Autodesk Inventor part; units mm, degrees
ref_plane "YZ Plane" through (0, 0, 0) normal (1, 0, 0) x (0, 1, 0)
ref_plane "XZ Plane" through (0, 0, 0) normal (0, 1, 0) x (-1, 0, 0)
ref_plane "XY Plane" through (0, 0, 0) normal (0, 0, 1) x (1, 0, 0)
sketch "Sketch1" plane through (0, 0, 0) normal (0, 1, 0) x (-1, 0, 0)
  line L0 (0, 0) -> (0, -35)
  line L1 (0, -35) -> (37, -35)
  line L2 (37, -35) -> (37, -55)
  line L3 (37, -55) -> (48, -55)
  line L4 (48, -55) -> (48, 0)
  line L5 (48, 0) -> (22, 0)
  line L6 (22, 0) -> (22, 0)
  line L7 (22, 0) -> (0, 0)
  dimension "d0" = 35
  dimension "d1" = 37
  dimension "d2" = 20
  dimension "d3" = 11
  dimension "d4" = 55
  dimension "d5" = 26
  dimension "d6" = 0
extrude "Extrusion1" add sketch "Sketch1" along normal blind 50
shell "Shell1" thickness 5 removed faces 3 at (-48, 16.6667, -36.6667) at (-19.6667, 0, -23.3333) at (-19.6667, 50, -23.3333)
sketch "Sketch2" plane through (0, 0, 0) normal (1, 0, 0) x (0, 0, -1)
  line L0 (5, 0) -> (30, 0)
  line L1 (5, 0) -> (19, 0)
  line L2 (19, 0) -> (19, 17)
  line L3 (19, 17) -> (5, 17)
  line L4 (5, 17) -> (5, 0)
  point P0 (0, 0)
  dimension "d10" = 17
  dimension "d11" = 0
  dimension "d12" = 11
extrude "Extrusion2" cut sketch "Sketch2" against normal blind 10
sketch "Sketch3" plane through (-48, 0, -55) normal (-1, 0, 0) x (0, 0, 1)
  line L0 (0, 0) -> (0, 50)
  line L1 (5, 50) -> (25, 50)
  line L2 (0, 0) -> (5, 0)
  line L3 (5, 0) -> (5, 50)
  line L4 (5, 50) -> (0, 50)
  line L5 (0, 50) -> (0, 0)
  point P0 (55, 0)
extrude "Extrusion3" add sketch "Sketch3" along normal blind 15
sketch "Sketch4" plane through (-48, 0, 0) normal (-1, 0, 0) x (0, 0, 1)
  line L0 (-5, 0) -> (0, 0)
  line L1 (-5, 0) -> (-5, 50)
  line L2 (0, 0) -> (-5, 0)
  line L3 (-5, 0) -> (-5, 50)
  line L4 (-5, 50) -> (0, 50)
  line L5 (0, 50) -> (0, 0)
  point P0 (0, 0)
extrude "Extrusion4" add sketch "Sketch4" along normal blind 15
sketch "Sketch5" plane through (0, 17, -5) normal (0, 0, -1) x (-1, 0, 0)
  circle A0 centre (11.5, -8.5) radius 2.0828
  line L0 (63, -17) -> (0, -17)
  line L1 (0, -17) -> (0, 0)
  dimension "d19" = 4.1656
  dimension "d20" = 8.5
  dimension "d21" = 11.5
extrude "Extrusion5" cut sketch "Sketch5" against normal blind 15
sketch "Sketch6" plane through (0, 17, -5) normal (0, 0, -1) x (-1, 0, 0)
  circle A0 centre (28.505, 18.46) radius 2.0828
  line L0 (63, -17) -> (0, -17)
  line L1 (5, 0) -> (5, 33)
  dimension "d24" = 4.1656
  dimension "d25" = 35.46
  dimension "d26" = 23.505
extrude "Extrusion6" cut sketch "Sketch6" against normal blind 15
sketch "Sketch7" plane through (0, 17, -5) normal (0, 0, -1) x (-1, 0, 0)
  circle A0 centre (58.5, 19) radius 2.0828
  line L0 (63, 33) -> (63, -17)
  line L1 (5, 33) -> (63, 33)
  point P0 (0, -17)
  dimension "d29" = 4.1656
  dimension "d30" = 4.5
  dimension "d31" = 14
extrude "Extrusion7" cut sketch "Sketch7" against normal blind 15
sketch "Sketch13" plane through (0, 0, -35) normal (0, 0, -1) x (-1, 0, 0)
  circle A0 centre (11.5, 8.5) radius 2.0828
  line L0 (0, 0) -> (37, 0)
  line L1 (0, 0) -> (0, 50)
  dimension "d41" = 4.1656
  dimension "d42" = 8.5
  dimension "d43" = 11.5
extrude "Extrusion9" cut sketch "Sketch13" against normal blind 15
sketch "Sketch14" plane through (-37, 0, -55) normal (0, 0, -1) x (-1, 0, 0)
  circle A0 centre (-8.495, 35.46) radius 2.0828
  line L0 (-37, 0) -> (-37, 50)
  line L1 (0, 0) -> (26, 0)
  dimension "d46" = 4.1656
  dimension "d47" = 28.505
  dimension "d48" = 35.46
extrude "Extrusion10" cut sketch "Sketch14" against normal blind 15
sketch "Sketch15" plane through (-37, 0, -55) normal (0, 0, -1) x (-1, 0, 0)
  circle A0 centre (21.5, 36) radius 2.0828
  line L0 (0, 0) -> (26, 0)
  line L1 (26, 50) -> (26, 0)
  point P0 (-37, 0)
  dimension "d51" = 4.1656
  dimension "d52" = 36
  dimension "d53" = 4.5
extrude "Extrusion11" cut sketch "Sketch15" against normal blind 15
sketch "Sketch16" plane through (-42, 0, -30) normal (-1, 0, 0) x (0, 0, 1)
  line L0 (0, 0) -> (-5, 0)
  line L1 (-5, 0) -> (-5, 50)
  line L2 (-5, 50) -> (0, 50)
  line L3 (0, 50) -> (0, 0)
  point P0 (30, 0)
  dimension "d56" = 5
  dimension "d57" = 50
extrude "Extrusion12" add sketch "Sketch16" along normal blind 21
sketch "Sketch17" plane through (-5, 0, -30) normal (0, 0, 1) x (1, 0, 0)
  circle A0 centre (-23.505, 35.46) radius 2.0828
  line L0 (0, 0) -> (0, 50)
  line L1 (0, 0) -> (-58, 0)
  point P0 (5, 0)
  dimension "d60" = 4.1656
  dimension "d61" = 23.505
  dimension "d62" = 35.46
extrude "Extrusion13" cut sketch "Sketch17" against normal blind 10
sketch "Sketch18" plane through (-42, 0, -35) normal (0, 0, -1) x (-1, 0, 0)
  circle A0 centre (16.5, 36) radius 2.0828
  line L0 (21, 50) -> (21, 0)
  line L1 (0, 0) -> (21, 0)
  point P0 (-42, 0)
  dimension "d65" = 4.1656
  dimension "d67" = 36
  dimension "d70" = 4.5
extrude "Extrusion14" cut sketch "Sketch18" against normal blind 10
sketch "Sketch20" plane through (-63, 0, 0) normal (-1, 0, 0) x (0, 0, 1)
  line L0 (0, 0) -> (-5, 0)
  line L1 (-5, 17) -> (-5, 50)
  line L2 (0, 0) -> (-5, 0)
  line L3 (-5, 0) -> (-5, 50)
  line L4 (-5, 50) -> (0, 50)
  line L5 (0, 50) -> (0, 0)
extrude "Extrusion15" add sketch "Sketch20" along normal blind 2.583
sketch "Sketch21" plane through (-63, 0, -30) normal (-1, 0, 0) x (0, 0, 1)
  line L0 (-20, 50) -> (-5, 50)
  line L1 (11, 0) -> (0, 0)
  line L2 (-5, 50) -> (0, 50)
  line L3 (0, 50) -> (0, 0)
  line L4 (0, 0) -> (-5, 0)
  line L5 (-5, 0) -> (-5, 50)
  point P0 (30, 0)
extrude "Extrusion16" add sketch "Sketch21" along normal blind 2.583
sketch "Sketch22" plane through (-63, 0, -55) normal (-1, 0, 0) x (0, 0, 1)
  line L0 (0, 0) -> (0, 50)
  line L1 (5, 0) -> (5, 50)
  line L2 (0, 50) -> (5, 50)
  line L3 (5, 50) -> (5, 0)
  line L4 (5, 0) -> (0, 0)
  line L5 (0, 0) -> (0, 50)
  point P0 (55, 0)
extrude "Extrusion17" add sketch "Sketch22" along normal blind 2.583
sketch "Sketch23" plane through (0, 0, 0) normal (0, 0, 1) x (1, 0, 0)
  line L0 (0, 50) -> (-37, 50)
  line L1 (-65.583, 50) -> (-65.583, 0)
  line L2 (0, 50) -> (-65.583, 50)
  line L3 (-65.583, 50) -> (-65.583, 43.083)
  line L4 (-65.583, 43.083) -> (0, 43.083)
  line L5 (0, 43.083) -> (0, 50)
  point P0 (0, 0)
  dimension "d77" = 6.917
extrude "Extrusion18" cut sketch "Sketch23" against normal blind 100
sketch "Sketch24" plane through (0, 0, -35) normal (0, 0, -1) x (-1, 0, 0)
  line L0 (0, 0) -> (65.583, 0)
  line L1 (31.0052, 0) -> (26.0052, 0)
  line L2 (26.0052, 5) -> (31.0052, 5)
  circle A0 centre (28.505, 35.46) radius 2.0828
  line L3 (26.0052, 5) -> (25.0052, 5)
  line L4 (25.0052, 5) -> (26.0052, 0)
  line L5 (31.0052, 5) -> (32.0052, 5)
  line L6 (32.0052, 5) -> (31.0052, 0)
  dimension "d80" = 5
  dimension "d81" = 5
  dimension "d83" = 1
  dimension "d84" = 1
extrude "Extrusion19" cut sketch "Sketch24" against normal blind 100 contours L4 L3 L2 L5 L6 L0
sketch "Sketch25" plane through (0, 0, 0) normal (1, 0, 0) x (0, 0, -1)
  line L0 (0, 0) -> (5, 0)
  line L1 (35, 43.083) -> (0, 43.083)
  line L2 (0, 0) -> (5, 0)
  line L3 (5, 0) -> (5, 43.083)
  line L4 (5, 43.083) -> (0, 43.083)
  line L5 (0, 43.083) -> (0, 0)
  dimension "d87" = 5
extrude "Extrusion20" cut sketch "Sketch25" against normal blind 100
sketch "Sketch26" plane through (0, 0, -19) normal (1, 0, 0) x (0, 0, -1)
  line L0 (-9, 35.6451) -> (-9, 26.9508)
  line L1 (-9, 26.9508) -> (-14, 27.8324)
  line L2 (-9, 35.6451) -> (-14, 34.7635)
  line L3 (-9, 35.6451) -> (-3.9229, 35.6451) construction
  line L4 (-14, 34.7635) -> (-14, 27.8324)
  line L5 (-14, 43.083) -> (-14, 17)
  line L6 (-14, 17) -> (0, 17)
  line L7 (16, 43.083) -> (-14, 43.083)
  point P0 (0, 0)
  dimension "d90" = 8.6943
  dimension "d91" = 80
  dimension "d92" = 170
  dimension "d93" = 0
  dimension "d94" = 5
  dimension "d128" = 7.4379
extrude "Extrusion21" cut sketch "Sketch26" against normal blind 100
sketch "Sketch27" plane through (-37, 0, -35) normal (1, 0, 0) x (0, 0, -1)
  line L0 (5, 17) -> (5, 8.3057)
  line L1 (5, 8.3057) -> (0, 9.1873)
  line L2 (5, 17) -> (0, 16.1184)
  line L3 (5, 17) -> (10.0771, 17) construction
  line L4 (0, 16.1184) -> (0, 9.1873)
  line L5 (0, 0) -> (0, 43.083)
  line L6 (20, 43.083) -> (0, 43.083)
  dimension "d98" = 8.6943
  dimension "d99" = 80
  dimension "d100" = 170
  dimension "d102" = 5
  dimension "d104" = 0
  dimension "d105" = 26.083
sketch "Sketch28" plane through (-37, 0, -35) normal (1, 0, 0) x (0, 0, -1)
  line L0 (5, 34.3887) -> (5, 25.6944)
  line L1 (5, 25.6944) -> (0, 26.576)
  line L2 (5, 34.3887) -> (0, 33.507)
  line L3 (5, 34.3887) -> (10.0771, 34.3887) construction
  line L4 (0, 33.507) -> (0, 26.576)
  dimension "d106" = 8.6943
  dimension "d107" = 80
  dimension "d108" = 170
  dimension "d109" = 5
extrude "Extrusion22" add sketch "Sketch27" along normal blind 5
extrude "Extrusion23" add sketch "Sketch28" along normal blind 5
sketch "Sketch29" plane through (-65.583, 43.083, -30) normal (0, 1, 0) x (1, 0, 0)
  line L0 (33.583, 5) -> (28.583, 5)
  line L1 (0, 25) -> (28.583, 25)
  line L2 (28.583, 5) -> (0, 5)
  line L3 (0, 5) -> (0, 25)
  line L4 (0, 25) -> (28.583, 25)
  line L5 (28.583, 25) -> (28.583, 5)
  point P0 (65.583, -30)
extrude "Extrusion24" cut sketch "Sketch29" against normal blind 100
sketch "Sketch31" plane through (-65.583, 43.083, -30) normal (0, 0, 1) x (1, 0, 0)
  line L0 (60.583, -8.3195) -> (60.583, 0)
  line L1 (60.583, 0) -> (-3.7083, 0)
  line L2 (-3.7083, 0) -> (-3.7083, -46.9701)
  line L3 (-3.7083, -46.9701) -> (60.583, -46.9701)
  line L4 (60.583, -46.9701) -> (60.583, 0)
  point P0 (65.583, -43.083)
extrude "Extrusion25" cut sketch "Sketch31" against normal blind 100
sketch "Sketch32" plane through (0, 0, -35) normal (0, 0, -1) x (-1, 0, 0)
  line L0 (10, 34.3887) -> (10, 25.6944)
  line L1 (10, 25.6944) -> (5, 26.576)
  line L2 (10, 34.3887) -> (5, 33.507)
  line L3 (10, 34.3887) -> (15.0771, 34.3887) construction
  line L4 (5, 33.507) -> (5, 26.576)
  line L5 (5, 0) -> (5, 43.083)
  line L6 (5, 43.083) -> (0, 43.083)
  dimension "d120" = 8.6943
  dimension "d121" = 80
  dimension "d122" = 170
  dimension "d123" = 5
  dimension "d124" = 0
  dimension "d125" = 8.6943
extrude "Extrusion26" add sketch "Sketch32" against normal blind 5
sketch "Sketch33" plane through (0, 0, -19) normal (1, 0, 0) x (0, 0, -1)
  line L0 (0, 0) -> (16, 0)
  line L1 (16, 0) -> (-15.3687, 0)
  line L2 (-15.3687, 0) -> (-15.3687, 22.832)
  line L3 (-15.3687, 22.832) -> (16, 22.832)
  line L4 (16, 22.832) -> (16, 0)
  point P0 (-19, 0)
  dimension "d130" = 22.832
extrude "Extrusion27" cut sketch "Sketch33" against normal blind 10
sketch "Sketch34" plane through (-10, 25.6944, -35) normal (-1, 0, 0) x (0, 0, 1)
  line L0 (0, -2.8624) -> (30, -2.8624)
  line L1 (0, 17.3886) -> (30, 17.3886)
  line L2 (0, -2.8624) -> (5, -2.8624)
  line L3 (5, -2.8624) -> (5, 17.3886)
  line L4 (5, 17.3886) -> (0, 17.3886)
  line L5 (0, 17.3886) -> (0, -2.8624)
  point P0 (35, -25.6944)
  dimension "d133" = 5
extrude "Extrusion28" add sketch "Sketch34" against normal blind 5
sketch "Sketch35" plane through (0, 43.083, -35) normal (0, 0, -1) x (-1, 0, 0)
  line L0 (10, -20.251) -> (10, 0)
  line L1 (10, -16.507) -> (14.9999, -17.3886)
  line L2 (10, -16.507) -> (15.077, -16.507) construction
  line L3 (14.9999, -17.3886) -> (14.9999, -8.6944)
  line L4 (14.9999, -8.6944) -> (10, -9.576)
  line L5 (10, -9.576) -> (10, -16.507)
  point P0 (0, -43.083)
  dimension "d136" = 5.077
  dimension "d137" = 10
  dimension "d138" = 5.077
  dimension "d139" = 3.744
  dimension "d140" = 6.931
extrude "Extrusion29" add sketch "Sketch35" against normal blind 5
properties part number "Frame VG01-2"
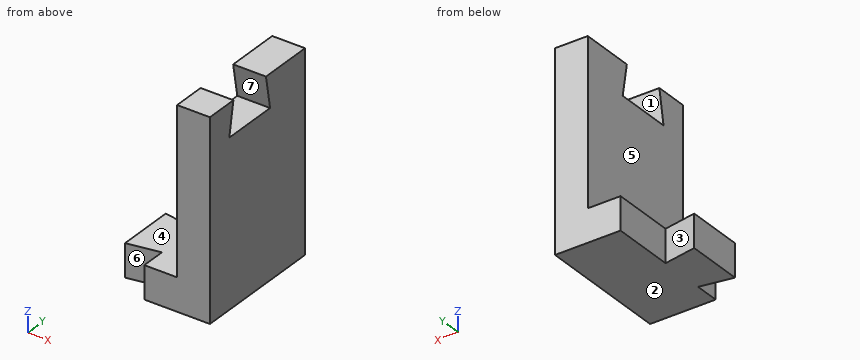
Input: part model. Units: mm. Frame: model coordinates. Face numbers are marked on the shaded views. A direction names the side the tool comes from. Give positions to 0.01 mm unless a question says otherwise; leave off trailing zeros. Write each loop counter-clockwise with the first axis right and the second up, starting at its lowest first coordinate (ties: lowest second). Pieces come first, ordered by that corner, then holes. Notation, with made-up numbers: M 81,-8 L 135,-8 A15 ccw 135,3 Z; hole C 27,-23.75 d3. An arc over 180 degrees is marked long. Write item = value, one per line. Start each with the question number.
1) Cut plane B-B on y = 38. Return the cut outline in (x, z).
2) Cut plane D-D on y = 26.25. Return the cut outline in (x, z), then the cut area to 3 significant figures.
3) Reachability of the marked faces 5, 6 and 7 from +Z, -Z, +X, -X, +Y, -Y: full face, straight path, thin tool, end or side. Return the list, or none.
4) Draft query along Z for the marked faces 1, 2, 3 and 4. Return one class per face: +Z half, -Z half, draft (parallel to the pull), parting line (faces both ways), or undercut.
5) First-contact query: pin 1 Ø1.9 at (y, z) = (24, -33) entering from -X; pin 2 Ø1.5 at (y, z) = (34.5, -17) entering from -X; pin 3 Ø3 at (x, y) = (-5.5, 30) entering from +Z; pin 4 Ø5 at (x, z) = (-8.5, -23.5) entering from -Y. Flat tips, straight axial feed; report the tip coordinate or a pass-through.
6) Material intervals for line 1 along Z through (x, y) = (-13, 31.75); line 2 along X through (y, z) = (40.5, -30.5); line 3 along X through (y, z) = (40.75, -10.5), sorted ascending. Write a range as [from, to].
7) Cut plane C-C on z = -30.5. Return the cut outline in (x, y).
8) Cut plane A-A on x = -3. Return the cut outline in (y, z), then the cut area to 3 significant figures.
Solved:
q1.outline = M -10,-35 L 0,-35 L 0,-5 L -5,-5 L -5,-30 L -10,-30 Z
q2.outline = M -15,-35 L -11.85,-35 L -11.85,-30 L -15,-30 Z; M -10,-35 L 0,-35 L 0,-5 L -5,-5 L -5,-30 L -10,-30 Z
q2.area = 191 mm2
q3.face_5 = +Z, -X, +Y, -Y
q3.face_6 = +Z, -Z, -Y
q3.face_7 = +X, -X
q4.face_1 = undercut
q4.face_2 = -Z half
q4.face_3 = draft
q4.face_4 = +Z half
q5.pin_1 = -10
q5.pin_2 = -5
q5.pin_3 = -10
q5.pin_4 = through
q6.line_1 = [-35, -30]
q6.line_2 = [-10, 0]
q6.line_3 = [-5, 0]
q7.outline = M -15,25.69 L -10,26.58 L -10,22.83 L 0,22.83 L 0,43.08 L -10,43.08 L -10,33.51 L -15,34.39 Z
q8.outline = M 22.83,-35 L 43.08,-35 L 43.08,-5 L 34.76,-5 L 35.65,-10 L 26.95,-10 L 27.83,-5 L 22.83,-5 Z
q8.area = 568 mm2
